Could you check a few things on this drawing? It's one solid part, dimensions in mm from its lowest x, y, z. Give positions to 0.01 mm unless a question says otherwise; leave off trailing zeros. Order: outer loops, then holes, each group sorted by start corner. A loop starts at its lowest first (then second) coordinate and runs counter-clockwise, first axis right, second up.
Item 1: I want a section at B-B, the plane y = 7.62. Write out the boundary of the cut face in (x, z).
Item 2: I want a section at D-D, the plane x = 62. Write out the boundary of the cut face in (y, z).
Item 3: I'm going to push a flat-ended pin straight in: pin 1 Ø23 at (x, y) = (57.5, 22.5) entering from -Z. Where does the tip first touch, or does it pass through?
Item 4: I want a section at C-C, the plane x = 12.7. Write out the boundary of the cut face in (y, z), then the cut area to 3 significant figures.
Item 5: If we mould it in two halves opening along Y, with no side actions, what happens to the marked faces 1 and 2? For each: +Y half, -Y half, draft (parallel to the pull), parting line (faces both ways), or undercut.
Item 6: I want a section at A-A, the plane z = 1.25. Write out the boundary of the cut face in (x, y).
Item 7: If I drill on line 1 along Y through (x, z) = (12.7, 5.5); line 2 along X through (y, z) = (7.62, 3.8); line 3 along Y through (x, z) = (76.5, 2.25), over which ranges is the centre line in solid material (lowest first)?
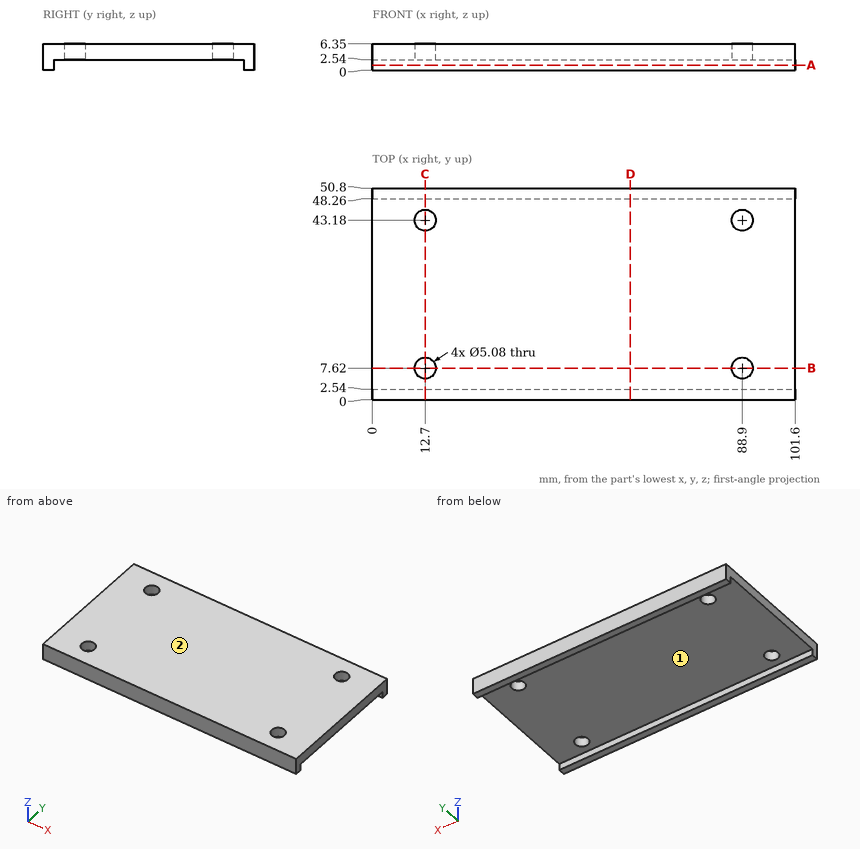
Results list:
1. outline: (0, 2.54) - (10.16, 2.54) - (10.16, 6.35) - (0, 6.35) - close; (15.24, 2.54) - (86.36, 2.54) - (86.36, 6.35) - (15.24, 6.35) - close; (91.44, 2.54) - (101.6, 2.54) - (101.6, 6.35) - (91.44, 6.35) - close
2. outline: (0, 0) - (2.54, 0) - (2.54, 2.54) - (48.26, 2.54) - (48.26, 0) - (50.8, 0) - (50.8, 6.35) - (0, 6.35) - close
3. pin 1: stops at z = 2.54
4. outline: (0, 0) - (2.54, 0) - (2.54, 2.54) - (5.08, 2.54) - (5.08, 6.35) - (0, 6.35) - close; (10.16, 2.54) - (40.64, 2.54) - (40.64, 6.35) - (10.16, 6.35) - close; (45.72, 2.54) - (48.26, 2.54) - (48.26, 0) - (50.8, 0) - (50.8, 6.35) - (45.72, 6.35) - close
4. area: 168 mm2
5. face 1: undercut
5. face 2: draft
6. outline: (0, 0) - (101.6, 0) - (101.6, 2.54) - (0, 2.54) - close; (0, 48.26) - (101.6, 48.26) - (101.6, 50.8) - (0, 50.8) - close
7. line 1: y = 0 to 5.08, 10.16 to 40.64, 45.72 to 50.8
7. line 2: x = 0 to 10.16, 15.24 to 86.36, 91.44 to 101.6
7. line 3: y = 0 to 2.54, 48.26 to 50.8
